Design review of the part shown in the three views and the two pictorial views. Dimensions are in mm from the part's minimum x, y and z. A direction names the side the tool comes from. Round coordinates to 2 decimals unless told otherwise and drop trailing zeros. Loops run counter-clockwise (first coordinate to the right, second up) from the corner with the lowest first, then second, coordinate; pieces in that order, holes last. Notation, with made-up numbers: M 30,63.25 L 68,63.25 A29 cw 68,99.25 Z; hole C -22,-17 d11. An arc over 180 degrees is marked long. Return JSON: item names as keys, results as strings. Group by question number.
Q1. For the marked faces 1 and 2, list the 3-axis set-ups (+Z, -Z, +X, -X, +Y, -Y) from which the entire face can be reached by the end or side of a thin tool; tool diameter is ignored.
Q2. Consider section C-C (z = 2). State the section outline as (x, y) points, and give its area (3 significant figures).
Q3. Consider section D-D (x = 14.25). State the section outline as (y, z) points.
Q4. Consider section A-A (y = 8). State the section outline as (x, z) points.
Q5. Consider section B-B (x = 19). State the section outline as (y, z) points.
Q6. Clearance check with flat-ended pins moving along their axes: pin 1 Ø5 at (x, z) = (3.5, 7) entering from +Y; pin 2 Ø9 at (x, z) = (13, 13) entering from +Y; pin 3 Ø4 at (x, z) = (21.082, 9.017) entering from -Y; pin 4 Ø5.5 at (y, z) = (9.144, 9.017) entering from +X. State where each tip first meets the part, or that it passes through.
Q7. To check wall thickness, follow line 1 along X through (y, z) = (18, 14.5); line 2 along Y through (x, z) = (2, 13.75). State the ranges of each line that lie inside material, in increasing order.
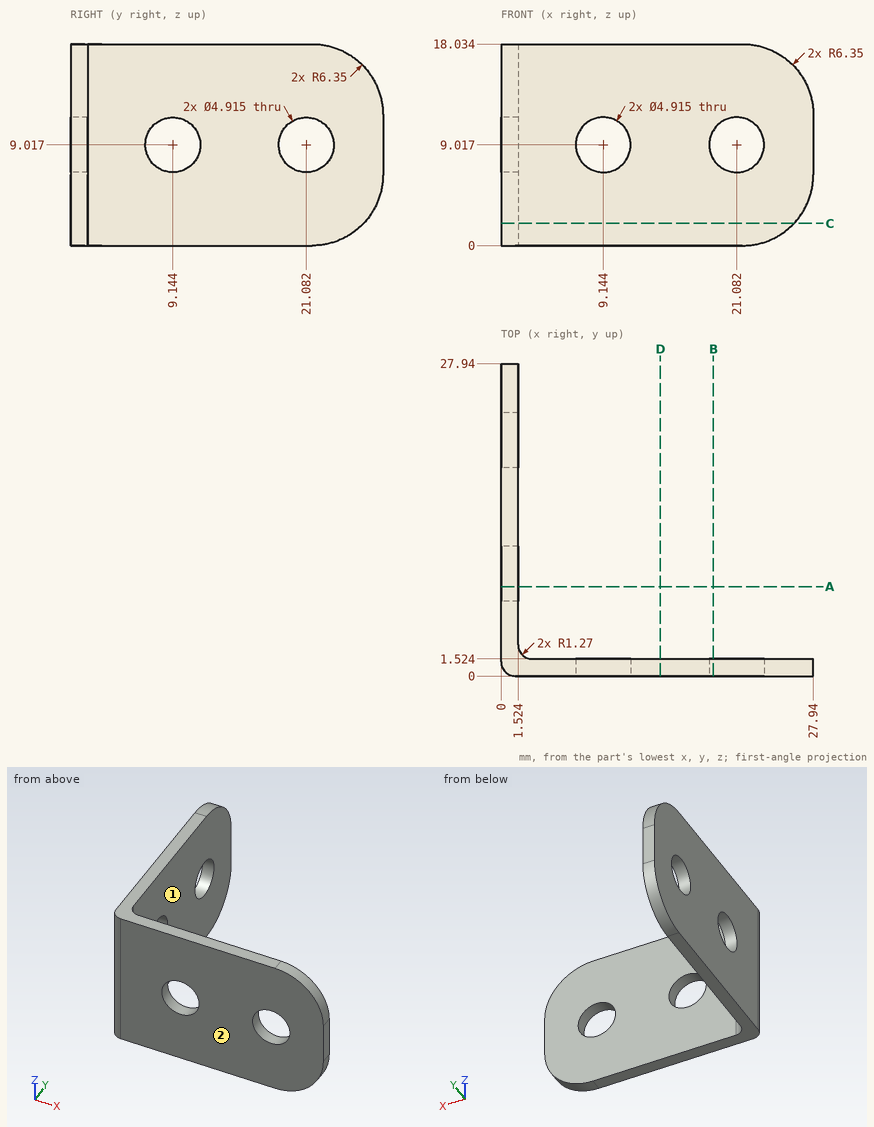
Values:
{
 "1": {"face 1": "+Z, -Z, +X, +Y", "face 2": "+Z, -Z, +X, -X, -Y"},
 "2": {"outline": "M 0,1.27 A1.27 ccw 1.27,0 L 26.22,0 L 26.22,1.52 L 2.79,1.52 A1.27 cw 1.52,2.79 L 1.52,26.22 L 0,26.22 Z", "area": "77.6 mm2"},
 "3": {"outline": "M 0,0 L 1.52,0 L 1.52,18.03 L 0,18.03 Z"},
 "4": {"outline": "M 0,0 L 1.52,0 L 1.52,6.84 L 0,6.84 Z; M 0,11.19 L 1.52,11.19 L 1.52,18.03 L 0,18.03 Z"},
 "5": {"outline": "M 0,0 L 1.52,0 L 1.52,7.71 L 0,7.71 Z; M 0,10.32 L 1.52,10.32 L 1.52,18.03 L 0,18.03 Z"},
 "6": {"pin 1": "stops at y = 27.94", "pin 2": "stops at y = 1.52", "pin 3": "passes through", "pin 4": "stops at x = 1.52"},
 "7": {"line 1": "x = 0 to 1.52", "line 2": "y = 0 to 1.8"}
}
